Could you check a few things on this model? Use its own coordinates, in mm. A direction names the side the tool comes from. Give positions to 0.01 mm unless a question says otherwise; leave off trailing zeros. Order: outer loops, then holes, each group sorted by start corner. A loop starts at its lowest first (then second) coordinate and runs counter-clockwise, first axis right, second up. Notation, with made-up numbers: M -30.5,-10.5 L 10.5,-10.5 A7 ccw 10.5,-5.5 Z; hole C -24,-31.75 d2. An arc over 180 degrees is marked long. Answer in a Markdown table with one row per item. Add a question column.
Autodesk Inventor part; units mm, degrees
ref_plane "YZ Plane" through (0, 0, 0) normal (1, 0, 0) x (0, 1, 0)
ref_plane "XZ Plane" through (0, 0, 0) normal (0, 1, 0) x (-1, 0, 0)
ref_plane "XY Plane" through (0, 0, 0) normal (0, 0, 1) x (1, 0, 0)
sketch "Sketch1" plane through (0, 0, 0) normal (1, 0, 0) x (0, 1, 0)
  line L0 (0, 0) -> (35, 0)
  line L1 (35, 0) -> (35, -50)
  line L2 (35, -50) -> (0, -50)
  line L3 (0, -50) -> (0, 0)
  line L4 (17.5, 0) -> (17.5, 11.9434)
  line L5 (19, 0) -> (19, 5)
  line L6 (16, 0) -> (16, 5)
  line L7 (-1, 5) -> (34, 5)
  line L8 (34, 5) -> (34, 15)
  line L9 (34, 15) -> (-1, 15)
  line L10 (-1, 15) -> (-1, 5)
  line L11 (16, 5) -> (19, 5)
  line L12 (19, 0) -> (16, 0)
  dimension "d0" = 35
  dimension "d1" = 50
  dimension "d2" = 5
  dimension "d3" = 1.5
  dimension "d4" = 1.5
  dimension "d11" = 10
  dimension "d12" = 0
extrude "Extrusion1" add sketch "Sketch1" along normal blind 5
sketch "Sketch3" plane through (5, 0, 0) normal (1, 0, 0) x (0, 0, -1)
  circle A0 centre (47.5, 17.5) radius 1.25
  line L0 (50, 0) -> (50, 35)
  line L1 (0, 0) -> (50, 0)
  dimension "d16" = 2.5
  dimension "d17" = 2.5
  dimension "d18" = 17.5
extrude "Extrusion3" cut sketch "Sketch3" against normal blind 5
equation "\"d3\" = 0.5 * Snap"
equation "\"d4\" = 0.5 * Snap"
equation "\"Snap\" = 3"
properties part number "Stresstest"
1. Suppose I cut it at C-C on x = 0.95. List the corners of the cut face in (y, z) for me.
2. Thinking about a two-plate mould opening in Z: for faces 1 (the flat face through (5, 17, -17)), 2 (the flat face through (2, 18, -50)), 3 (the flat face through (2, 16, 2)), which applies, pulls with the +Z half, pulls with the -Z half, needs draft (parallel to the pull), parting line crosses it, or undercut?
3. Will these pins go through, and if not, where does the flat tip stop? P1, Ø2.5, axis at x = 3, z = 2, coming from the +Y side; P2, Ø1, axis at x = 1.5, z = -11, coming from the -Y side; P3, Ø3, axis at x = 4, z = 2.5, coming from the -Y side.
4. For faces 4 (the flat face through (2, 0, -25)), 5 (the flat face through (2, 27, 0)), 6 (the flat face through (2, 8, 0)), which set-ups out of +Z, -Z, +X, -X, +Y, -Y let a thin tool reach every point of the face, with its end or its side?
5. If I drill on line 1 along Z through (x, y) = (3.15, 4); line 2 along Y through (x, z) = (1.4, -47.5); line 3 along Y through (x, z) = (4.85, 5.5), over which ranges is the centre line in solid material (lowest first)? Write a range as [from, to].
6. Suppose I cut it at B-B on z = -47.5. List the corners of the cut face in (x, y) for me, plus the area to 4 significant figures.
7. Suppose I cut it at A-A on y = 17.5. List the corners of the cut face in (x, z) for me, plus the area to 4 significant figures.
8. Suppose I cut it at D-D on z = -17. List the corners of the cut face in (x, y) for me.
Findings below:
| question | item | result |
|---|---|---|
| 1 | outline | M -1,5 L 16,5 L 16,0 L 0,0 L 0,-50 L 35,-50 L 35,0 L 19,0 L 19,5 L 34,5 L 34,15 L -1,15 Z; hole C 17.5,-47.5 d2.5 |
| 2 | face 1 | needs draft |
| 2 | face 2 | pulls with the -Z half |
| 2 | face 3 | undercut |
| 3 | P1 | y = 19 |
| 3 | P2 | y = 0 |
| 3 | P3 | y = 16 |
| 4 | face 4 | -Z, +X, -X, -Y |
| 4 | face 5 | +X, -X, +Y |
| 4 | face 6 | +X, -X, -Y |
| 5 | line 1 | [-50, 0], [5, 15] |
| 5 | line 2 | [0, 16.25], [18.75, 35] |
| 5 | line 3 | [-1, 34] |
| 6 | outline | M 0,0 L 5,0 L 5,16.25 L 0,16.25 Z; M 0,18.75 L 5,18.75 L 5,35 L 0,35 Z |
| 6 | area | 162.5 mm2 |
| 7 | outline | M 0,-50 L 5,-50 L 5,-48.75 L 0,-48.75 Z; M 0,-46.25 L 5,-46.25 L 5,15 L 0,15 Z |
| 7 | area | 312.5 mm2 |
| 8 | outline | M 0,0 L 5,0 L 5,35 L 0,35 Z |
